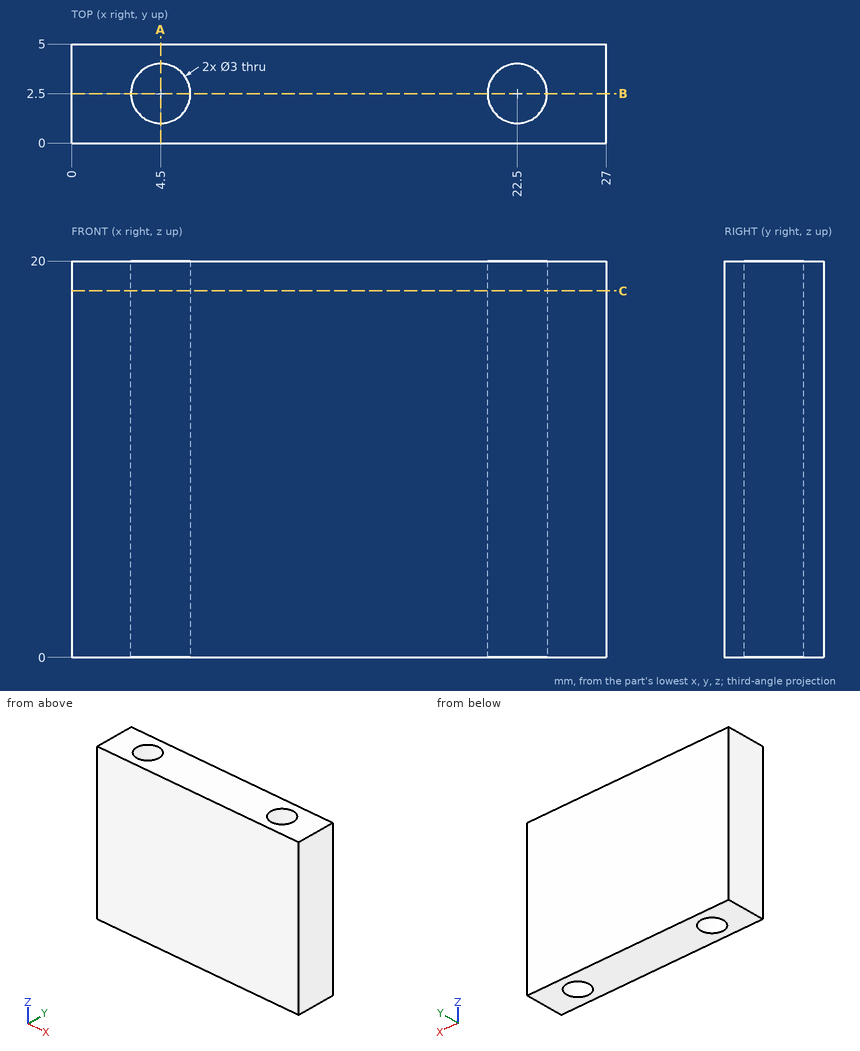
Job drawing, mm, ordinate dimensions from the low corner. One solid piece. Coordinates: 2 decimals unless noted, no trailing zeros. Write each loop counter-clockwise with the first axis right and the second up, starting at its lowest first coordinate (ties: lowest second). Pieces come first, ordered by that corner, then holes. Notation, with made-up numbers: (20, -8.5) - (34, -8.5) arc R24 cw to (34, 29.5) - close; hole circle Ø11 at (43, -18.5). An arc over 180 degrees is marked (long way). Use a Markdown table: item, result. Add a question column.
Item 1: Drill centre lines: L1, parallel to X at y = 2.6, z = 6.5; L2, parallel to Y at x = 22.5, z = 12; L3, parallel to X at y = 1.4, z = 15.25. Where is each one in solid material? Low to high. Write a range as from..to.
Item 2: Band-saw the part on C-C, the plane z = 18.5. Give the cut face in (x, y).
Item 3: Band-saw the part on A-A, the plane x = 4.5. Give the cut face in (y, z), and give its area (3 significant figures).
Item 4: Flat gauge pin, fed straight in: pin 1 (1.8 mm diameter, centred on x = 22.5, y = 2.5, fed in from +Z). Where does the tip first touch, or does it go through?
Item 5: Band-saw the part on B-B, the plane y = 2.5. Give the cut face in (x, z).
Numbers:
| question | item | result |
|---|---|---|
| 1 | L1 | 0..3, 6..21, 24..27 |
| 1 | L2 | 0..1, 4..5 |
| 1 | L3 | 0..3.48, 5.52..21.48, 23.52..27 |
| 2 | outline | (0, 0) - (27, 0) - (27, 5) - (0, 5) - close; hole circle Ø3 at (4.5, 2.5); hole circle Ø3 at (22.5, 2.5) |
| 3 | outline | (0, 0) - (1, 0) - (1, 20) - (0, 20) - close; (4, 0) - (5, 0) - (5, 20) - (4, 20) - close |
| 3 | area | 40.0 mm2 |
| 4 | pin 1 | through |
| 5 | outline | (0, 0) - (3, 0) - (3, 20) - (0, 20) - close; (6, 0) - (21, 0) - (21, 20) - (6, 20) - close; (24, 0) - (27, 0) - (27, 20) - (24, 20) - close |
